Autodesk Fusion 360 part; units mm, degrees
sketch "Sketch1" plane through (0, 0, 0) normal (0, 1, 0) x (1, 0, 0)
  line L0 (0, 0) -> (90, 0)
  line L1 (90, 0) -> (90, 90)
  line L2 (90, 90) -> (0, 90)
  line L3 (0, 90) -> (0, 0)
  dimension "d1" = 90
  dimension "d2" = 90
extrude "Extrude1" add sketch "Sketch1" along normal blind 11
sketch "Sketch2" plane through (0, 11, 0) normal (0, 1, 0) x (-1, 0, 0)
  line L0 (0, -90) -> (0, 0)
  line L1 (0, 0) -> (-90, 0)
  line L2 (-90, 0) -> (-90, -90)
  line L3 (-90, -90) -> (0, -90)
  circle A0 centre (-5, -85) radius 3.875
  circle A1 centre (-5, -5) radius 3.875
  circle A2 centre (-85, -5) radius 3.875
  circle A3 centre (-85, -85) radius 3.875
  dimension "d5" = 7.75
  dimension "d6" = 7.75
  dimension "d7" = 7.75
  dimension "d8" = 7.75
extrude "Extrude2" cut sketch "Sketch2" against normal blind 4.5 contours A0 | A1 | A2 | A3
sketch "Sketch3" plane through (0, 11, 0) normal (0, 1, 0) x (-1, 0, 0)
  circle A0 centre (-85, -85) radius 3.875
  circle A1 centre (-5, -5) radius 3.875
  circle A2 centre (-5, -85) radius 3.875
  circle A3 centre (-85, -5) radius 3.875
  line L0 (0, -90) -> (0, 0)
  line L1 (0, 0) -> (-90, 0)
  line L2 (-90, 0) -> (-90, -90)
  line L3 (-90, -90) -> (0, -90)
  line L4 (-90, -80) -> (-90, -10)
  line L5 (0, -10) -> (0, -80)
  line L6 (-10, -90) -> (-80, -90)
  line L7 (-80, 0) -> (-10, 0)
  line L8 (-10, 0) -> (-10, -7)
  line L9 (-10, -83) -> (-10, -90)
  line L10 (-90, -10) -> (-83, -10)
  line L11 (-7, -10) -> (0, -10)
  line L12 (-80, -90) -> (-80, -83)
  line L13 (-80, -7) -> (-80, 0)
  line L14 (0, -80) -> (-7, -80)
  line L15 (-83, -80) -> (-90, -80)
  line L16 (0, -10) -> (-3, -10)
  line L17 (-3, -10) -> (-3, -30)
  line L18 (-3, -30) -> (0, -30)
  line L19 (0, -30) -> (0, -10)
  line L20 (0, -80) -> (-3, -80)
  line L21 (-3, -80) -> (-3, -60)
  line L22 (-3, -60) -> (0, -60)
  line L23 (0, -60) -> (0, -80)
  line L24 (-10, -90) -> (-30, -90)
  line L25 (-30, -90) -> (-30, -87)
  line L26 (-30, -87) -> (-10, -87)
  line L27 (-10, -87) -> (-10, -90)
  line L28 (-80, -90) -> (-60, -90)
  line L29 (-60, -90) -> (-60, -87)
  line L30 (-60, -87) -> (-80, -87)
  line L31 (-80, -87) -> (-80, -90)
  line L32 (-90, -80) -> (-87, -80)
  line L33 (-87, -80) -> (-87, -60)
  line L34 (-87, -60) -> (-90, -60)
  line L35 (-90, -60) -> (-90, -80)
  line L36 (-90, -10) -> (-87, -10)
  line L37 (-87, -10) -> (-87, -30)
  line L38 (-87, -30) -> (-90, -30)
  line L39 (-90, -30) -> (-90, -10)
  line L40 (-80, 0) -> (-60, 0)
  line L41 (-60, 0) -> (-60, -3)
  line L42 (-60, -3) -> (-80, -3)
  line L43 (-80, -3) -> (-80, 0)
  line L44 (-10, 0) -> (-30, 0)
  line L45 (-30, 0) -> (-30, -3)
  line L46 (-30, -3) -> (-10, -3)
  line L47 (-10, -3) -> (-10, 0)
  arc A4 (-10, -7) -> (-7, -10) centre (-7, -7) ccw
  arc A5 (-83, -10) -> (-80, -7) centre (-83, -7) ccw
  arc A6 (-80, -83) -> (-83, -80) centre (-83, -83) ccw
  arc A7 (-7, -80) -> (-10, -83) centre (-7, -83) ccw
  dimension "d11" = 20
  dimension "d12" = 3
  dimension "d13" = 20
  dimension "d14" = 3
  dimension "d15" = 20
  dimension "d16" = 3
  dimension "d17" = 20
  dimension "d18" = 3
  dimension "d19" = 3
  dimension "d20" = 20
  dimension "d21" = 3
  dimension "d22" = 20
  dimension "d23" = 3
  dimension "d24" = 20
  dimension "d25" = 20
  dimension "d26" = 3
  dimension "d27" = 3
  dimension "d28" = 3
extrude "Extrude3" cut sketch "Sketch3" against normal blind 8 contours L0 L1 L2 L3 L4 L5 L6 L7 L8 L9 L10 L11 L12 L13 L14 L15 L17 L18 L21 L22 L25 L26 L29 L30 L33 L34 L37 L38 L41 L42 L45 L46 A4 A5 A6 A7
sketch "Sketch4" plane through (0, 3, 0) normal (0, 1, 0) x (-1, 0, 0)
  line L0 (-3, -80) -> (-3, -60)
  line L1 (-3, -60) -> (0, -60)
  line L2 (0, -60) -> (0, -30)
  line L3 (0, -30) -> (-3, -30)
  line L4 (-3, -30) -> (-3, -10)
  line L5 (-3, -10) -> (-7, -10)
  arc A0 (-10, -7) -> (-7, -10) centre (-7, -7) ccw
  line L6 (-10, -7) -> (-10, -3)
  line L7 (-10, -3) -> (-30, -3)
  line L8 (-30, -3) -> (-30, 0)
  line L9 (-30, 0) -> (-60, 0)
  line L10 (-60, 0) -> (-60, -3)
  line L11 (-60, -3) -> (-80, -3)
  line L12 (-80, -3) -> (-80, -7)
  arc A1 (-83, -10) -> (-80, -7) centre (-83, -7) ccw
  line L13 (-83, -10) -> (-87, -10)
  line L14 (-87, -10) -> (-87, -30)
  line L15 (-87, -30) -> (-90, -30)
  line L16 (-90, -30) -> (-90, -60)
  line L17 (-90, -60) -> (-87, -60)
  line L18 (-87, -60) -> (-87, -80)
  line L19 (-87, -80) -> (-83, -80)
  arc A2 (-80, -83) -> (-83, -80) centre (-83, -83) ccw
  line L20 (-80, -83) -> (-80, -87)
  line L21 (-80, -87) -> (-60, -87)
  line L22 (-60, -87) -> (-60, -90)
  line L23 (-60, -90) -> (-30, -90)
  line L24 (-30, -90) -> (-30, -87)
  line L25 (-30, -87) -> (-10, -87)
  line L26 (-10, -87) -> (-10, -83)
  arc A3 (-7, -80) -> (-10, -83) centre (-7, -83) ccw
  line L27 (-7, -80) -> (-3, -80)
  line L28 (0, -60) -> (-3, -60)
  line L29 (-3, -60) -> (-3, -30)
  line L30 (-3, -30) -> (0, -30)
  line L31 (0, -30) -> (0, -60)
  line L32 (-87, -30) -> (-90, -30)
  line L33 (-90, -30) -> (-90, -60)
  line L34 (-90, -60) -> (-87, -60)
  line L35 (-87, -60) -> (-87, -30)
  line L36 (-30, 0) -> (-60, 0)
  line L37 (-60, 0) -> (-60, -3)
  line L38 (-60, -3) -> (-30, -3)
  line L39 (-30, -3) -> (-30, 0)
  line L40 (-30, -90) -> (-60, -90)
  line L41 (-60, -90) -> (-60, -87)
  line L42 (-60, -87) -> (-30, -87)
  line L43 (-30, -87) -> (-30, -90)
extrude "Extrude4" add sketch "Sketch4" along normal blind 4 contours L1 L2 L3 L28 L29 L30 L31 | L22 L23 L24 L40 L41 L42 L43 | L8 L9 L10 L36 L37 L38 L39 | L15 L16 L17 L32 L33 L34 L35
fillet "Fillet1" radius 3 8 edges at (90, 5.5, 0) (90, 0, -45) (45, 0, 0) (90, 5.5, -90) (45, 0, -90) (0, 5.5, -90) (0, 0, -45) (0, 5.5, 0)
sketch "Sketch6" plane through (0, 3, 0) normal (0, 1, 0) x (-1, 0, 0)
  line L0 (-87, -10) -> (-87, -80)
  line L1 (-87, -80) -> (-83, -80)
  arc A0 (-80, -83) -> (-83, -80) centre (-83, -83) ccw
  line L2 (-80, -83) -> (-80, -87)
  line L3 (-80, -87) -> (-10, -87)
  line L4 (-10, -87) -> (-10, -83)
  arc A1 (-7, -80) -> (-10, -83) centre (-7, -83) ccw
  line L5 (-7, -80) -> (-3, -80)
  line L6 (-3, -80) -> (-3, -10)
  line L7 (-3, -10) -> (-7, -10)
  arc A2 (-10, -7) -> (-7, -10) centre (-7, -7) ccw
  line L8 (-10, -7) -> (-10, -3)
  line L9 (-10, -3) -> (-80, -3)
  line L10 (-80, -3) -> (-80, -7)
  arc A3 (-83, -10) -> (-80, -7) centre (-83, -7) ccw
  line L11 (-83, -10) -> (-87, -10)
  arc A4 (-3, -90) -> (0, -87) centre (-3, -87) ccw
  line L12 (0, -87) -> (0, -60)
sketch "Sketch7" plane through (45, 3, -45) normal (0, 1, 0) x (-1, 0, 0)
CAD build for the part. Positions are in the model's coordinates, mm. A direction names the side the tool comes from. Give positions to 0.01 mm unless a question says otherwise; leave off trailing zeros. Loops run counter-clockwise (first coordinate to the right, second up) from the corner with the lowest first, then second, coordinate; pieces in that order, holes last. Notation, with made-up numbers: M 73,38.25 L 107,38.25 A20 cw 107,62.25 Z; hole C 1.25,-29 d5. An arc over 180 degrees is marked long. Answer in a Markdown table with one row per item. Add a question column.
Item 1: Band-saw the part on D-D on y = 9.5. Give the number of separate pieces and of enclosed holes in the cut face, then the cut area to 3 significant figures.
Item 2: Probe probe 1 along Z at (x, y) = (5, 9.9) (3 decimals); probe 2 along Z at (x, y) = (68, 8.5); probe 3 along X at (y, z) = (10, -3.5). List the from-to ranges inside material, lowest first.
Item 3: Band-saw the part on B-B on x = 5. Give the cut face in (y, z) (3 decimals).
Item 4: Drop flat-ended pins along their axis: P1, Ø4.5, axis at x = 85, z = -85, coming from the +Y side; P2, Ø3.5, axis at y = 9.5, z = -1, coming from the +X side; P3, Ø0.9, axis at x = 50, z = -1.5, coming from the +Y side. Give the stop position or say it passes through.
Item 5: Tool access for faces 1 (the face through (88.87, 8.78, -4.83)), 2 (the face through (89, 7, -45)), 3 (the face through (45, 7, -1)): list every direction of +Z, -Z, +X, -X, +Y, -Y with a clear straight run to the whole face (end or side of a thin tool).
Item 6: Band-saw the part on C-C on z = -51. Give the cut face in (x, y), then the cut area to 3 significant figures.
Item 7: Band-saw the part on A-A on y = 4.25. Give the cut face in (x, z).
Item 8: Mould opens along Z. For faces 4 (the face through (85, 6.5, -85)), 5 (the face through (89.14, 7.06, -89.1)), 6 (the face through (0.86, 0.9, -44.41)) say: +Z half, -Z half, draft (parallel to the pull), parting line (faces both ways), or undercut.
Reply:
| question | item | result |
|---|---|---|
| 1 | separate pieces | 4 |
| 1 | enclosed holes | 4 |
| 1 | area | 676 mm^2 |
| 2 | probe 1 | z = -90 to -88.875, -81.125 to -80, -10 to -8.875, -1.125 to 0 |
| 2 | probe 2 | z = -90 to -87, -3 to 0 |
| 2 | probe 3 | x = 0 to 1.43, 8.57 to 10, 80 to 81.43, 88.57 to 90 |
| 3 | outline | M 0,-87 A3 ccw 3,-90 L 11,-90 L 11,-88.875 L 6.5,-88.875 L 6.5,-81.125 L 11,-81.125 L 11,-80 L 3,-80 L 3,-10 L 11,-10 L 11,-8.875 L 6.5,-8.875 L 6.5,-1.125 L 11,-1.125 L 11,0 L 3,0 A3 ccw 0,-3 Z |
| 4 | P1 | stops at y = 6.5 |
| 4 | P2 | stops at x = 89.99 |
| 4 | P3 | stops at y = 7 |
| 5 | face 1 | +Y |
| 5 | face 2 | +X, -X, +Y |
| 5 | face 3 | +Z, -Z, +Y |
| 6 | outline | M 0,3 A3 ccw 3,0 L 87,0 A3 ccw 90,3 L 90,7 L 87,7 L 87,3 L 3,3 L 3,7 L 0,7 Z |
| 6 | area | 290 mm^2 |
| 7 | outline | M 0,-87 A3 ccw 3,-90 L 87,-90 A3 ccw 90,-87 L 90,-3 A3 ccw 87,0 L 3,0 A3 ccw 0,-3 Z; hole M 3,-80 L 7,-80 A3 cw 10,-83 L 10,-87 L 80,-87 L 80,-83 A3 cw 83,-80 L 87,-80 L 87,-10 L 83,-10 A3 cw 80,-7 L 80,-3 L 10,-3 L 10,-7 A3 cw 7,-10 L 3,-10 Z |
| 8 | face 4 | undercut |
| 8 | face 5 | -Z half |
| 8 | face 6 | draft |
